```python
from build123d import *

# Parameters (mm, degrees)
SKETCH1_W           = 96
SKETCH1_H           = 66
BOSS_EXTRUDE2_DEPTH = 3
SKETCH4_R           = 2
BOSS_EXTRUDE3_DEPTH = 3
SKETCH8_R           = 2.5
BOSS_EXTRUDE5_DEPTH = 3.5
SKETCH9_W           = 96
SKETCH9_H           = 66
SKETCH9_W_2         = 87.5
SKETCH9_H_2         = 58.2
BOSS_EXTRUDE6_DEPTH = 18
SKETCH11_W          = 54
SKETCH11_H          = 14
CUT_EXTRUDE1_DEPTH  = 4
SKETCH12_W          = 43
SKETCH12_H          = 3.5
CUT_EXTRUDE2_DEPTH  = 4.5
SKETCH13_W          = 16
SKETCH13_H          = 5
CUT_EXTRUDE3_DEPTH  = 3.5
SKETCH14_R          = 4
SKETCH14_W          = 12
SKETCH14_H          = 8.5
SKETCH14_W_2        = 20
SKETCH14_H_2        = 10
CUT_EXTRUDE4_DEPTH  = 2.3
SKETCH16_R          = 2
BOSS_EXTRUDE7_DEPTH = 18
CHAMFER2_SIZE       = 1


with BuildPart() as part:
    # Sketch1 → Boss-Extrude2 (new body)
    with BuildSketch(Plane(origin=(0, 0, 0), x_dir=(1, 0, 0), z_dir=(0, 1, 0))):
        Rectangle(SKETCH1_W, SKETCH1_H)
    extrude(amount=BOSS_EXTRUDE2_DEPTH)

    # Sketch4 → Boss-Extrude3 (add)
    # profile 1 of 3: a face of its own
    with BuildSketch(Plane(origin=(0, 0, 0), x_dir=(1, 0, 0), z_dir=(0, 1, 0))):
        with BuildLine():
            Line((-43, 33), (-43, 39.5))
            ThreePointArc((-43, 39.5), (-38, 44.5), (-33, 39.5))
            Line((-33, 39.5), (-33, 33))
            ThreePointArc((-33, 33), (-38, 28), (-43, 33))
        make_face()
        with Locations(Location((-38, 39.5, 0), (0, 0, 270))):
            Circle(SKETCH4_R, mode=Mode.SUBTRACT)
    # profile 2 of 3: a face of its own
    with BuildSketch(Plane(origin=(0, 0, 0), x_dir=(1, 0, 0), z_dir=(0, 1, 0))):
        with BuildLine():
            Line((-28, -33), (-28, -39.5))
            ThreePointArc((-28, -39.5), (-33, -44.5), (-38, -39.5))
            Line((-38, -39.5), (-38, -33))
            ThreePointArc((-38, -33), (-33, -28), (-28, -33))
        make_face()
        with Locations(Location((-33, -39.5, 0), (0, 0, 270))):
            Circle(SKETCH4_R, mode=Mode.SUBTRACT)
    # profile 3 of 3: a face of its own
    with BuildSketch(Plane(origin=(0, 0, 0), x_dir=(1, 0, 0), z_dir=(0, 1, 0))):
        with BuildLine():
            Line((38, -33), (38, -39.5))
            ThreePointArc((38, -39.5), (33, -44.5), (28, -39.5))
            Line((28, -39.5), (28, -33))
            ThreePointArc((28, -33), (33, -28), (38, -33))
        make_face()
        with Locations(Location((33, -39.5, 0), (0, 0, 270))):
            Circle(SKETCH4_R, mode=Mode.SUBTRACT)
    extrude(amount=BOSS_EXTRUDE3_DEPTH)

    # Sketch8 → Boss-Extrude5 (add)
    with BuildSketch(Plane(origin=(0, 3, 0), x_dir=(1, 0, 0), z_dir=(0, 1, 0))):
        with Locations(Location((-19.25, 26.1, 0), (0, 0, 270))):
            Circle(SKETCH8_R)
        with Locations(Location((38.75, 26.1, 0), (0, 0, 270))):
            Circle(SKETCH8_R)
        with Locations(Location((38.75, -22.9, 0), (0, 0, 270))):
            Circle(SKETCH8_R)
        with Locations(Location((-19.25, -22.9, 0), (0, 0, 270))):
            Circle(SKETCH8_R)
    extrude(amount=BOSS_EXTRUDE5_DEPTH)

    # Sketch9 → Boss-Extrude6 (add)
    with BuildSketch(Plane(origin=(0, 3, 0), x_dir=(1, 0, 0), z_dir=(0, 1, 0))):
        Rectangle(SKETCH9_W, SKETCH9_H)
        with Locations((-0.25, 1.6)):
            Rectangle(SKETCH9_W_2, SKETCH9_H_2, mode=Mode.SUBTRACT)
    extrude(amount=BOSS_EXTRUDE6_DEPTH)

    # Sketch11 → Cut-Extrude1 (cut)
    with BuildSketch(Plane.ZY.offset(48)):
        with Locations((0, 14)):
            Rectangle(SKETCH11_W, SKETCH11_H)
    extrude(amount=-CUT_EXTRUDE1_DEPTH, mode=Mode.SUBTRACT)

    # Sketch12 → Cut-Extrude2 (cut)
    with BuildSketch(Plane(origin=(48, 0, 0), x_dir=(0, 0, -1), z_dir=(1, 0, 0))):
        with Locations((1.5, 19.25)):
            Rectangle(SKETCH12_W, SKETCH12_H)
    extrude(amount=-CUT_EXTRUDE2_DEPTH, mode=Mode.SUBTRACT)

    # Sketch13 → Cut-Extrude3 (cut)
    with BuildSketch(Plane.ZY.offset(-43.5)):
        with Locations((-1.07504867, 5.5)):
            Rectangle(SKETCH13_W, SKETCH13_H)
    extrude(amount=-CUT_EXTRUDE3_DEPTH, mode=Mode.SUBTRACT)

    # Sketch14 → Cut-Extrude4 (cut)
    with BuildSketch(Plane(origin=(0, 0, -33), x_dir=(-1, 0, 0), z_dir=(0, 0, -1))):
        with Locations((10, 10.8)):
            Circle(SKETCH14_R)
        with Locations((-32.9, 9.05)):
            Rectangle(SKETCH14_W, SKETCH14_H)
        with Locations((-11.5, 11.1)):
            Rectangle(SKETCH14_W_2, SKETCH14_H_2)
    extrude(amount=-CUT_EXTRUDE4_DEPTH, mode=Mode.SUBTRACT)

    # Sketch16 → Boss-Extrude7 (add)
    # profile 1 of 3: a face of its own
    with BuildSketch(Plane(origin=(0, 3, 0), x_dir=(1, 0, 0), z_dir=(0, 1, 0))):
        with BuildLine():
            Line((-43, 33), (-33, 33))
            Line((-33, 33), (-33, 39.5))
            ThreePointArc((-33, 39.5), (-38, 44.5), (-43, 39.5))
            Line((-43, 39.5), (-43, 33))
        make_face()
        with Locations(Location((-38, 39.5, 0), (0, 0, 90))):
            Circle(SKETCH16_R, mode=Mode.SUBTRACT)
    # profile 2 of 3: a face of its own
    with BuildSketch(Plane(origin=(0, 3, 0), x_dir=(1, 0, 0), z_dir=(0, 1, 0))):
        with BuildLine():
            Line((-38, -33), (-38, -39.5))
            ThreePointArc((-38, -39.5), (-33, -44.5), (-28, -39.5))
            Line((-28, -39.5), (-28, -33))
            Line((-28, -33), (-38, -33))
        make_face()
        with Locations(Location((-33, -39.5, 0), (0, 0, 90))):
            Circle(SKETCH16_R, mode=Mode.SUBTRACT)
    # profile 3 of 3: a face of its own
    with BuildSketch(Plane(origin=(0, 3, 0), x_dir=(1, 0, 0), z_dir=(0, 1, 0))):
        with BuildLine():
            Line((28, -39.5), (28, -33))
            Line((28, -33), (38, -33))
            Line((38, -33), (38, -39.5))
            ThreePointArc((38, -39.5), (33, -44.5), (28, -39.5))
        make_face()
        with Locations(Location((33, -39.5, 0), (0, 0, 90))):
            Circle(SKETCH16_R, mode=Mode.SUBTRACT)
    extrude(amount=BOSS_EXTRUDE7_DEPTH)

    # Chamfer2
    chamfer2_edges = [part.edges().sort_by_distance(p)[0] for p in [
        (-45.5, 0, -33),
        (-33, 0, -36.25),
        (-38, 0, -44.5),
        (-43, 0, -36.25),
        (-43, 0, 33),
        (-38, 0, 36.25),
        (-33, 0, 44.5),
        (-28, 0, 36.25),
        (0, 0, 33),
        (48, 0, 0),
        (28, 0, 36.25),
        (33, 0, 44.5),
        (38, 0, 36.25),
        (43, 0, 33),
        (-48, 0, 0),
        (7.5, 0, -33),
        (48, 10.5, -33),
        (48, 10.5, 33),
        (-48, 10.5, 33),
        (-48, 10.5, -33),
    ]]
    chamfer(chamfer2_edges, length=CHAMFER2_SIZE)


solid = part.part
```
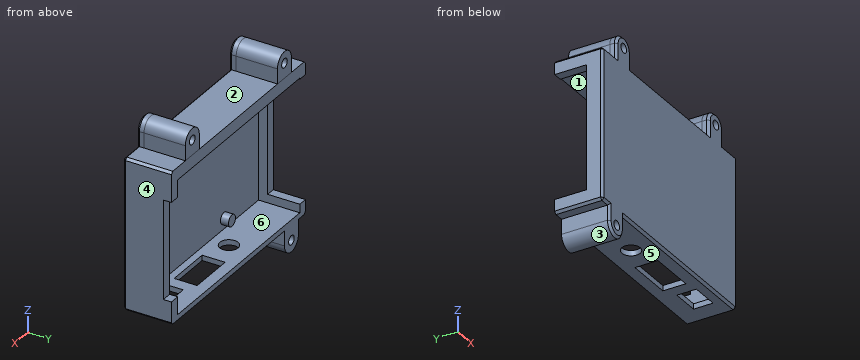
Source: CAD feature listing. Evaluate the final solid. Frame: model axes, mm. Face numbers are marked on the shaded views. A direction names the side the tool comes from. Coordinates: 2 decimals unless noted, no trailing zeros. Loops run counter-clockwise (first coordinate to the right, second up) from the corner with the lowest first, then second, coordinate; pieces in that order, holes last. Notation, with made-up numbers: (55, 82.25) - (95, 82.25) arc R19 ccw to (95, 118.25) - close; hole circle Ø6 at (6.5, 26). An arc over 180 degrees is marked (long way). Answer as CSV lines item,"result".
1. Reachability of the marked faces 4, 5 and 6 from +Z, -Z, +X, -X, +Y, -Y: full face, straight path, thin tool, end or side. Return the list, or none.
Established:
face 4,"+Z, -Z, +X, +Y, -Y"
face 5,"-Z, +X, +Y, -Y"
face 6,"+Y"
2. Section A-A (x = -10). Return loops of the section in (y, z), then the cut area to 3 significant figures.
Established:
outline,"(0, -32) - (1, -33) - (6.8, -33) - (6.8, -30.7) - (3, -30.7) - (3, 27.5) - (21, 27.5) - (21, 33) - (1, 33) - (0, 32) - close; (14.8, -33) - (21, -33) - (21, -30.7) - (14.8, -30.7) - close"
area,"319 mm2"
3. Section C-C (x = 10). Return loops of the section in (y, z), then the cut area to 3 significant figures.
Established:
outline,"(0, -32) - (1, -33) - (6.1, -33) - (6.1, -30.7) - (3, -30.7) - (3, 27.5) - (21, 27.5) - (21, 33) - (1, 33) - (0, 32) - close; (16.1, -33) - (21, -33) - (21, -30.7) - (16.1, -30.7) - close"
area,"314 mm2"
4. Contact query for flat-ended pins moving along their axis: pin 1 (2.5 mm diameter, centred on x = -42, y = 13, fed in from +Z); pin 2 (10 mm diameter, centred on x = -22, y = 4.5, fed in from -Z); pin 3 (1 mm diameter, centred on y = 12, z = 4, fed in from -X). Output: stop coordinate, or through.
Established:
pin 1,"stops at z = 33"
pin 2,"stops at z = -33"
pin 3,"stops at x = 43.5"
5. Section B-B (z = -2). Return loops of the section in (x, y).
Established:
outline,"(-48, 1) - (-47, 0) - (47, 0) - (48, 1) - (48, 17.5) - (43.5, 17.5) - (43.5, 8) - (47, 8) - (47, 3) - (-44, 3) - (-44, 7) - (-48, 7) - close"
6. Section D-D (z = -13). Return loops of the section in (x, y).
Established:
outline,"(-48, 1) - (-47, 0) - (47, 0) - (48, 1) - (48, 17.5) - (43.5, 17.5) - (43.5, 3) - (-44, 3) - (-44, 7) - (-48, 7) - close"
7. Ray query, line 1 (X direction, y = 1.35, z = 39.5); line 2 (Z direction, x = 8, y = 18.75); line 3 (X direction, y = 8.75, z = 35.5). Return the intervals inside material, ascending.
Established:
line 1,"x = -38 to -35, -31 to -28, 28 to 31, 35 to 38"
line 2,"z = -33 to -30.7, 27.5 to 33"
line 3,"x = -38 to -28, 28 to 38"
8. Mould query, pull axis Z, two halves, no side actions, for the marked faces 1, 2 and 3. Classes: released by +Z, released by -Z, zero draft, split by the parting line, or undercut.
Established:
face 1,"undercut"
face 2,"released by +Z"
face 3,"released by -Z"
